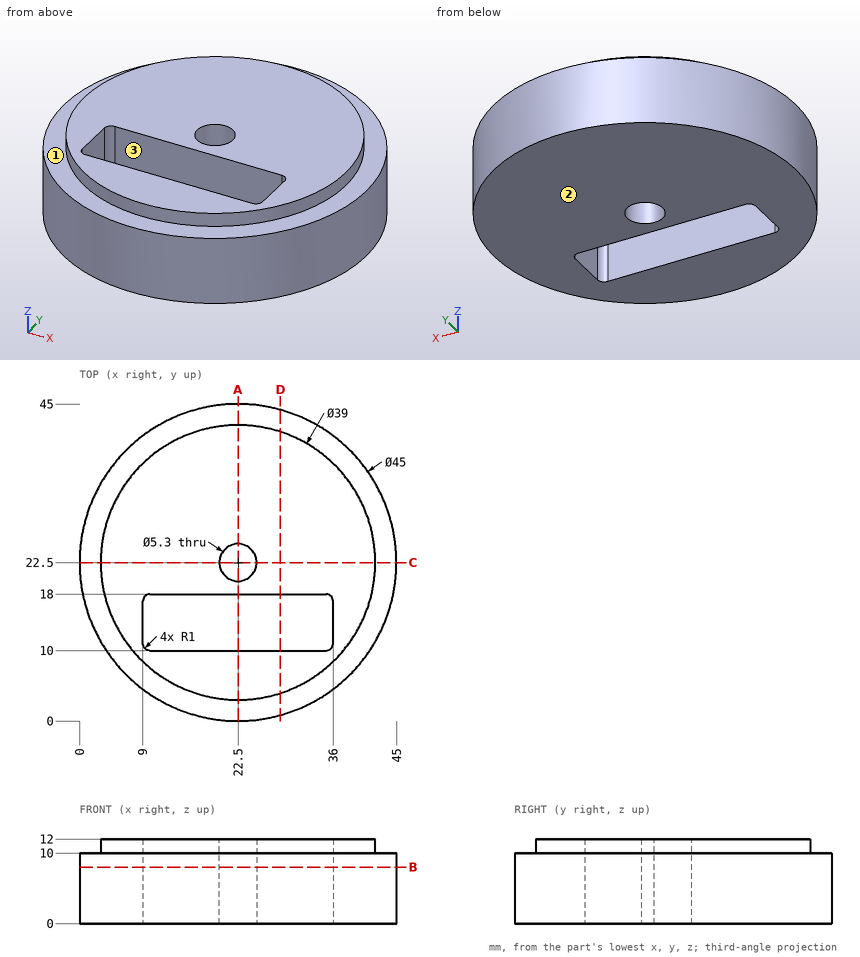
Source: three-view drawing plus pictorial views. Frame: mm from the lowest corner of the part. A direction names the side the tool comes from. Give positions to 0.01 mm unless a question says otherwise; leave off trailing zeros. Order: outer loops, then holes, each group sorted by start corner. A loop starts at its lowest first (then second) coordinate and runs counter-clockwise, first axis right, second up. Notation, with made-up numbers: (-25, 24) - (-11, 24) arc R37 ccw to (-11, 62) - close; hole circle Ø4 at (37, 16.25). An arc over 180 degrees is marked (long way). Answer as a JSON object with one key per item and string values. Group by question number.
Q1. Line query: probe 1 along Y at (x, z) = (22.5, 3); probe 2 along Y at (x, z) = (20.5, 11.75); probe 3 along Z at (x, y) = (42, 15). Output: solid intervals per line, ascending.
Q2. Cut plane D-D, the plane x = 28.5. Output: boundary loops of the cut face in (y, z).
Q3. Set-up query: the marked faces 1, 2 and 3. Return all of +Z, -Z, +X, -X, +Y, -Y with unobstructed straight access to the full face (end or side cutting, diameter ignored); none if empty.
Q4. First-contact query: pin 1 Ø1 at (y, z) = (19, 5.5) entering from -X; pin 2 Ø5 at (y, z) = (15, 5.5) entering from +X; pin 3 Ø1.5 at (y, z) = (11.5, 2.5) entering from +X; pin 4 Ø3 at (x, y) = (22.5, 22.5) entering from +Z. Flat tips, straight axial feed; report the tip coordinate or a pass-through.
Q5. Cut plane C-C, the plane y = 22.5. Output: boundary loops of the cut face in (x, z), then the cut area to 3 significant figures.
Q6. Cut plane B-B, the plane z = 8. Output: boundary loops of the cut face in (x, y), then the cut area to 3 significant figures.
Q7. Cut plane A-A, the plane x = 22.5. Output: boundary loops of the cut face in (y, z).
Results:
{
 "1": {"probe 1": "0 to 10, 18 to 19.85, 25.15 to 45", "probe 2": "3.1 to 10, 18 to 20.76, 24.24 to 41.9", "probe 3": "0 to 10"},
 "2": {"outline": "(0.81, 0) - (10, 0) - (10, 12) - (3.95, 12) - (3.95, 10) - (0.81, 10) - close; (18, 0) - (44.19, 0) - (44.19, 10) - (41.05, 10) - (41.05, 12) - (18, 12) - close"},
 "3": {"face 1": "+Z", "face 2": "-Z, +X, -X, +Y, -Y", "face 3": "+Z, -Z"},
 "4": {"pin 1": "x = 0.2", "pin 2": "x = 44.44", "pin 3": "x = 42.53", "pin 4": "through"},
 "5": {"outline": "(0, 0) - (19.85, 0) - (19.85, 12) - (3, 12) - (3, 10) - (0, 10) - close; (25.15, 0) - (45, 0) - (45, 10) - (42, 10) - (42, 12) - (25.15, 12) - close", "area": "464 mm^2"},
 "6": {"outline": "circle Ø45 at (22.5, 22.5); hole (9, 11) arc R1 ccw to (10, 10) - (35, 10) arc R1 ccw to (36, 11) - (36, 17) arc R1 ccw to (35, 18) - (10, 18) arc R1 ccw to (9, 17) - close; hole circle Ø5.3 at (22.5, 22.5)", "area": "1,350 mm^2"},
 "7": {"outline": "(0, 0) - (10, 0) - (10, 12) - (3, 12) - (3, 10) - (0, 10) - close; (18, 0) - (19.85, 0) - (19.85, 12) - (18, 12) - close; (25.15, 0) - (45, 0) - (45, 10) - (42, 10) - (42, 12) - (25.15, 12) - close"}
}
